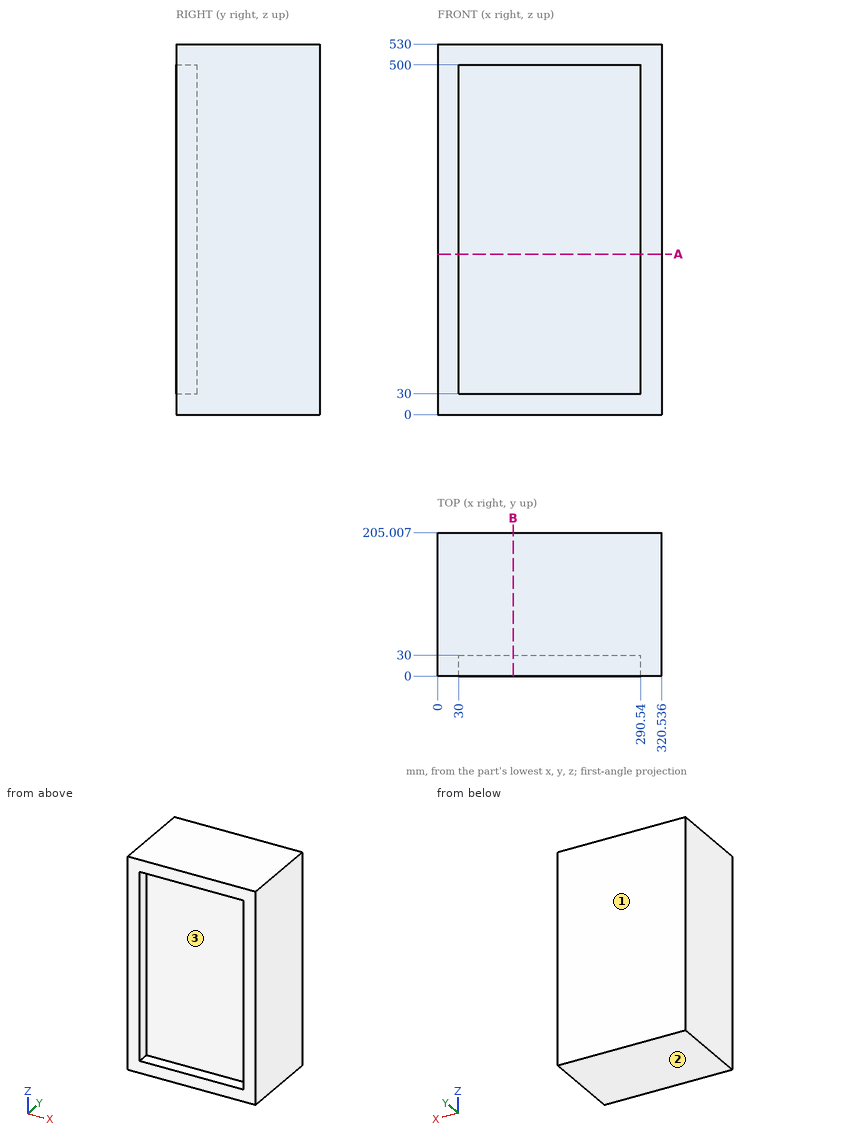
Drawing for the job (mm, zero at the part's lowest x, y, z). Round coordinates to 2 decimals unless told otherwise and drop trailing zeros. Write each loop counter-clockwise with the first axis right and the second up, starting at its lowest first coordinate (ties: lowest second). Pieces come first, ordered by that corner, then holes.
Item 1: Band-saw the part on B-B on x = 108. Write the cut outline in (y, z), then the cut area to 3 significant figures.
Filled in:
outline: (0, 0) - (205.01, 0) - (205.01, 530) - (0, 530) - (0, 500) - (30, 500) - (30, 30) - (0, 30) - close
area: 94,600 mm2
Item 2: Drill centre lines: L1, parallel to Z at x = 286, y = 11.5; L2, parallel to X at y = 19, z = 43.5 (1 decimal); L3, parallel to Y at x = 42, z = 177.5. Where is each one in solid material? Low to high.
Filled in:
L1: z = 0 to 30, 500 to 530
L2: x = 0 to 30, 290.5 to 320.5
L3: y = 30 to 205.01
Item 3: Band-saw the part on A-A on z = 229.5. Write the cut outline in (x, y) (1 decimal).
Filled in:
outline: (0, 0) - (30, 0) - (30, 30) - (290.5, 30) - (290.5, 0) - (320.5, 0) - (320.5, 205) - (0, 205) - close
Item 4: Drop a flat-ended pin along its axis: pin 1 Ø3 at (x, z) = (169.5, 435) entering from -Y. Give the stop position or say it passes through.
Filled in:
pin 1: stops at y = 30
Item 5: Mould opens along Z. For the marked faces 1, 2 and 3 say: released by +Z, released by -Z, zero draft, split by the parting line, or undercut.
Filled in:
face 1: zero draft
face 2: released by -Z
face 3: undercut
